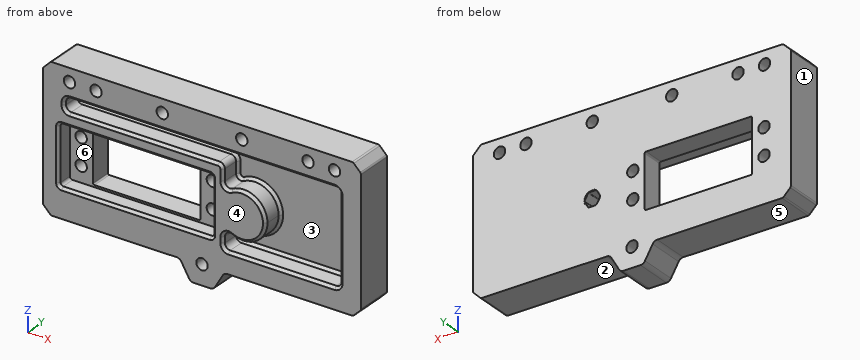
```python
from build123d import *

# Parameters (mm, degrees)
SKETCH_1_W          = 120
SKETCH_1_H          = 44
SKETCH_1_R          = 2.15
EXTRUDE_1_DEPTH     = 8
SKETCH_2_R          = 3
CUT_EXTRUDE_1_DEPTH = 0.1
MOVE_FACE_1_BY      = 10
EXTRUDE_START       = 6
SKETCH_3_W          = 120
SKETCH_3_H          = 54
SKETCH_3_W_2        = 58
SKETCH_3_H_2        = 22
EXTRUDE_2_DEPTH     = 6
SKETCH_4_R          = 2.15
CUT_EXTRUDE_2_DEPTH = 92.942930669
CUT_EXTRUDE_3_DEPTH = 8
FILLET_1_R          = 2
FILLET_2_R          = 2
FILLET_4_R          = 1
CHAMFER_1_SIZE      = 3
FILLET_5_R          = 1
SKETCH_6_R          = 2.15
EXTRUDE_3_DEPTH     = 14
SKETCH_6_3_R        = 2.15
CUT_EXTRUDE_6_DEPTH = 92.942930669
FILLET_6_R          = 2
CHAMFER_2_SIZE      = 1
SKETCH1_R           = 5.281314446
BOSS_EXTRUDE1_DEPTH = 4
SKETCH_7_R          = 2.15
CUT_EXTRUDE_7_DEPTH = 92.942930669


with BuildPart() as part:
    # 草图1 → 凸台-拉伸1 (new body)
    with BuildSketch(Plane(origin=(0, 0, 0), x_dir=(1, 0, 0), z_dir=(0, 1, 0))):
        with Locations((25.05, 0)):
            Rectangle(SKETCH_1_W, SKETCH_1_H)
        with Locations(Location((-24.75, 5, 0), (0, 0, 270))):
            Circle(SKETCH_1_R, mode=Mode.SUBTRACT)
        with Locations(Location((-24.75, -5, 0), (0, 0, 270))):
            Circle(SKETCH_1_R, mode=Mode.SUBTRACT)
        with Locations(Location((24.75, -5, 0), (0, 0, 270))):
            Circle(SKETCH_1_R, mode=Mode.SUBTRACT)
        with Locations(Location((24.75, 5, 0), (0, 0, 270))):
            Circle(SKETCH_1_R, mode=Mode.SUBTRACT)
        with BuildLine():
            Line((19.75, -10.25), (-19.75, -10.25))
            ThreePointArc((-19.75, -10.25), (-20.103553391, -10.103553391), (-20.25, -9.75))
            Line((-20.25, -9.75), (-20.25, 9.75))
            ThreePointArc((-20.25, 9.75), (-20.103553391, 10.103553391), (-19.75, 10.25))
            Line((-19.75, 10.25), (19.75, 10.25))
            ThreePointArc((19.75, 10.25), (20.103553391, 10.103553391), (20.25, 9.75))
            Line((20.25, 9.75), (20.25, -9.75))
            ThreePointArc((20.25, -9.75), (20.103553391, -10.103553391), (19.75, -10.25))
        make_face(mode=Mode.SUBTRACT)
        with BuildLine():
            Line((42.994486373, 0.15), (41.652146997, 2.475))
            ThreePointArc((41.652146997, 2.475), (41.542339376, 2.584807621), (41.392339376, 2.625))
            Line((41.392339376, 2.625), (38.707660624, 2.625))
            ThreePointArc((38.707660624, 2.625), (38.557660624, 2.584807621), (38.447853003, 2.475))
            Line((38.447853003, 2.475), (37.105513627, 0.15))
            ThreePointArc((37.105513627, 0.15), (37.065321248, 0), (37.105513627, -0.15))
            Line((37.105513627, -0.15), (38.447853003, -2.475))
            ThreePointArc((38.447853003, -2.475), (38.557660624, -2.584807621), (38.707660624, -2.625))
            Line((38.707660624, -2.625), (41.392339376, -2.625))
            ThreePointArc((41.392339376, -2.625), (41.542339376, -2.584807621), (41.652146997, -2.475))
            Line((41.652146997, -2.475), (42.994486373, -0.15))
            ThreePointArc((42.994486373, -0.15), (43.034678752, 0), (42.994486373, 0.15))
        make_face(mode=Mode.SUBTRACT)
    extrude(amount=EXTRUDE_1_DEPTH)

    # 草图2 → 切除-拉伸1 (cut)
    with BuildSketch(Plane(origin=(0, 8, 0), x_dir=(1, 0, 0), z_dir=(0, 1, 0))):
        with Locations(Location((40.05, 0, 0), (0, 0, 270))):
            Circle(SKETCH_2_R)
    extrude(amount=-CUT_EXTRUDE_1_DEPTH, mode=Mode.SUBTRACT)

    # Move Face 1: a face moved outward by 10.0
    extrude(part.faces().sort_by_distance((25.05, 4, 22))[0], amount=MOVE_FACE_1_BY, dir=(0, 0, 1))

    # 草图3 → 凸台-拉伸2 (add)
    with BuildSketch(Plane.XZ.offset(EXTRUDE_START)):
        with Locations((25.05, 5)):
            Rectangle(SKETCH_3_W, SKETCH_3_H)
        Rectangle(SKETCH_3_W_2, SKETCH_3_H_2, mode=Mode.SUBTRACT)
        with BuildLine():
            Line((41.652146997, 2.475), (42.994486373, 0.15))
            ThreePointArc((42.994486373, 0.15), (43.034678752, 0), (42.994486373, -0.15))
            Line((42.994486373, -0.15), (41.652146997, -2.475))
            ThreePointArc((41.652146997, -2.475), (41.542339376, -2.584807621), (41.392339376, -2.625))
            Line((41.392339376, -2.625), (38.707660624, -2.625))
            ThreePointArc((38.707660624, -2.625), (38.557660624, -2.584807621), (38.447853003, -2.475))
            Line((38.447853003, -2.475), (37.105513627, -0.15))
            ThreePointArc((37.105513627, -0.15), (37.065321248, 0), (37.105513627, 0.15))
            Line((37.105513627, 0.15), (38.447853003, 2.475))
            ThreePointArc((38.447853003, 2.475), (38.557660624, 2.584807621), (38.707660624, 2.625))
            Line((38.707660624, 2.625), (41.392339376, 2.625))
            ThreePointArc((41.392339376, 2.625), (41.542339376, 2.584807621), (41.652146997, 2.475))
        make_face(mode=Mode.SUBTRACT)
    extrude(amount=-EXTRUDE_2_DEPTH)

    # 草图4 → 切除-拉伸2 (cut, through all)
    with BuildSketch(Plane.XZ.offset(6)):
        with Locations(Location((-24.95, 27, 0), (0, 0, 270))):
            Circle(SKETCH_4_R)
        with Locations(Location((-14.95, 27, 0), (0, 0, 270))):
            Circle(SKETCH_4_R)
        with Locations(Location((65.05, 27, 0), (0, 0, 90))):
            Circle(SKETCH_4_R)
        with Locations(Location((75.05, 27, 0), (0, 0, 90))):
            Circle(SKETCH_4_R)
    extrude(amount=-CUT_EXTRUDE_2_DEPTH, mode=Mode.SUBTRACT)

    # 草图5 → 切除-拉伸3 (cut)
    with BuildSketch(Plane.XZ.offset(6)):
        with BuildLine():
            Line((59.05, 21), (-8.95, 21))
            Line((-8.95, 21), (-26.95, 21))
            Line((-26.95, 21), (-26.95, 16))
            Line((-26.95, 16), (33, 16))
            Line((33, 16), (33, 5.59441686))
            ThreePointArc((33, 5.59441686), (43.012262649, 8.498529285), (49.05, 0))
            ThreePointArc((49.05, 0), (43.012262649, -8.498529285), (33, -5.59441686))
            Line((33, -5.59441686), (33, -14))
            Line((33, -14), (77.05, -14))
            Line((77.05, -14), (77.05, 21))
            Line((77.05, 21), (59.05, 21))
        make_face()
    extrude(amount=-CUT_EXTRUDE_3_DEPTH, mode=Mode.SUBTRACT)

    # 圆角1
    fillet_1_edges = [part.edges().sort_by_distance(p)[0] for p in [
        (33, -2, 5.59441686),
        (33, -2, 16),
        (-26.95, -2, 16),
        (-26.95, -2, 21),
        (77.05, -2, 21),
        (77.05, -2, -14),
        (33, -2, -14),
    ]]
    fillet(fillet_1_edges, radius=FILLET_1_R)

    # 圆角2
    fillet_2_edges = [part.edges().sort_by_distance(p)[0] for p in [
        (33, -2, -5.59441686),
    ]]
    fillet(fillet_2_edges, radius=FILLET_2_R)

    # 圆角4
    fillet_4_edges = [part.edges().sort_by_distance(p)[0] for p in [
        (-29, -3, -11),
        (29, -3, -11),
        (29, -3, 11),
        (-29, -3, 11),
    ]]
    fillet(fillet_4_edges, radius=FILLET_4_R)

    # 倒角1
    chamfer_1_edges = [part.edges().sort_by_distance(p)[0] for p in [
        (-34.95, 1, -22),
        (85.05, 1, -22),
        (85.05, 1, 32),
        (-34.95, 1, 32),
    ]]
    chamfer(chamfer_1_edges, length=CHAMFER_1_SIZE)

    # 圆角5
    fillet_5_edges = [part.edges().sort_by_distance(p)[0] for p in [
        (85.05, 1, -19),
        (85.05, 1, 29),
        (-31.95, 1, 32),
        (82.05, 1, 32),
        (-31.95, 1, -22),
        (82.05, 1, -22),
        (-34.95, 1, -19),
        (-34.95, 1, 29),
    ]]
    fillet(fillet_5_edges, radius=FILLET_5_R)

    # 草图6 → 凸台-拉伸3 (add)
    with BuildSketch(Plane.XZ.offset(6)):
        Polygon((33.710254038, -21.5), (29.380127019, -14), (20.719872981, -14), (16.389745962, -21.5), (20.719872981, -29), (29.380127019, -29), align=None)
        with Locations((25.05, -21.5)):
            Circle(SKETCH_6_R, mode=Mode.SUBTRACT)
    extrude(amount=-EXTRUDE_3_DEPTH)

    # 草图6<3> → 切除-拉伸6 (cut, through all)
    with BuildSketch(Plane.XZ.offset(6)):
        with Locations(Location((25.05, -21.5, 0), (0, 0, 270))):
            Circle(SKETCH_6_3_R)
    extrude(amount=-CUT_EXTRUDE_6_DEPTH, mode=Mode.SUBTRACT)

    # 圆角6
    fillet_6_edges = [part.edges().sort_by_distance(p)[0] for p in [
        (16.678421097, 1, -22),
        (33.421578903, 1, -22),
        (20.719872981, 1, -29),
        (29.380127019, 1, -29),
    ]]
    fillet(fillet_6_edges, radius=FILLET_6_R)

    # 倒角2
    chamfer_2_edges = [part.edges().sort_by_distance(p)[0] for p in [
        (33, -6, 11.886141115),
        (33, 2, 11.886141115),
        (33, 2, -10.886141115),
        (55.025, 2, -14),
        (77.05, 2, 3.5),
        (25.05, 2, 21),
        (-26.95, 2, 18.5),
        (3.025, 2, 16),
        (33.585786438, 2, -13.414213562),
        (-26.364213562, 2, 20.414213562),
        (76.464213562, 2, -13.414213562),
        (76.464213562, 2, 20.414213562),
        (-26.364213562, 2, 16.585786438),
        (33.95989511, 2, 8.06401357),
        (3.025, -6, 16),
        (-26.95, -6, 18.5),
        (25.05, -6, 21),
        (77.05, -6, 3.5),
        (55.025, -6, -14),
        (33, -6, -10.886141115),
        (32.414213562, -6, 15.414213562),
        (33.95989511, -6, 8.06401357),
        (-26.364213562, -6, 16.585786438),
        (76.464213562, -6, 20.414213562),
        (76.464213562, -6, -13.414213562),
        (-26.364213562, -6, 20.414213562),
        (33.585786438, -6, -13.414213562),
        (32.414213562, 2, 15.414213562),
        (49.05, 2, 0),
        (49.05, -6, 0),
        (33.95989511, 2, -8.06401357),
        (33.95989511, -6, -8.06401357),
        (0, -6, -11),
        (29, -6, 0),
        (0, -6, 11),
        (-29, -6, 0),
        (28.707106781, -6, -10.707106781),
        (28.707106781, -6, 10.707106781),
        (-28.707106781, -6, -10.707106781),
        (-28.707106781, -6, 10.707106781),
    ]]
    chamfer(chamfer_2_edges, length=CHAMFER_2_SIZE)

    # Sketch1 → Boss-Extrude1 (add)
    with BuildSketch(Plane.XZ.offset(6)):
        with Locations((40.074190607, 0)):
            Circle(SKETCH1_R)
    extrude(amount=-BOSS_EXTRUDE1_DEPTH)

    # 草图7 → 切除-拉伸7 (cut, through all)
    with BuildSketch(Plane.XZ.offset(6)):
        with Locations(Location((10.05, 27, 0), (0, 0, 270))):
            Circle(SKETCH_7_R)
        with Locations(Location((40.05, 27, 0), (0, 0, 90))):
            Circle(SKETCH_7_R)
    extrude(amount=-CUT_EXTRUDE_7_DEPTH, mode=Mode.SUBTRACT)


solid = part.part
```
The listing builds one solid part. Answer for the finished solid, in the listing's coordinates (mm). Face numbers are marked on the shaded views. A direction names the side the tool comes from. Coordinates: 2 decimals unless noted, no trailing zeros. Loops run counter-clockwise (first coordinate to the right, second up) from the corner with the lowest first, then second, coordinate; pieces in that order, holes last. Notation, with made-up numbers: M 48.25,26.5 L 53.25,26.5 A17 ccw 53.25,40.5 Z; hole C 69,80 d3. An arc over 180 degrees is marked long. Answer as a JSON object with one key per item and string values. Group by question number.
Item 1: Which of the six approach directions +Z, -Z, +X, -X, +Y, -Y give full straight-line access (tool end or side, diameter ignored) to the marked faces 1, 2 and 3?
Item 2: Each of these flat-tipped pins is pushed along its axis until it touches: P1, Ø4, axis at x = 51, y = 2, coming from the -Z side; P2, Ø5.5, axis at x = 40.05, z = 27, coming from the +Y side; P3, Ø3, axis at x = 40, z = 0, coming from the +Y side; P4, Ø5, axis at x = -24.75, z = -5, coming from the -Y side. Where does it stop, or does it pass through?
Item 3: Section C-C (x = -8) is taken. Write down the section's boundary in (y, z), and give its area (3 significant figures).
Item 4: Consider L1, parallel to X at y = 5, z = -5; L2, parallel to Z at x = 75.05, y = -1; L3, parallel to X at y = -1, z = -9.5. Determine where each line is inside the solid, lowest interval first.
Item 5: Section D-D (z = 5) is taken. Give the number of separate pieces and of enclosed holes in the cut face, and give its area (3 significant figures).
Item 6: Section B-B (z = 27) is taken. Write down the section's boundary in (x, y), and give its area (3 significant figures).
Item 7: Determine the mould class of the marked faces 4, 5 and 6 for opening direction Z: +Z half, -Z half, draft (parallel to the pull), parting line (faces both ways), or undercut.
Solved:
{
 "1": {"face 1": "+Z, -Z, -X, +Y, -Y", "face 2": "-Z, +X, +Y, -Y", "face 3": "-Y"},
 "2": {"P1": "stops at z = -22", "P2": "stops at y = 8", "P3": "stops at y = -2", "P4": "stops at y = 0"},
 "3": {"outline": "M -6,-22 L 8,-22 L 8,-10.25 L 0,-10.25 L 0,-11 L -5,-11 L -6,-12 Z; M -6,12 L -5,11 L 0,11 L 0,10.25 L 8,10.25 L 8,32 L -6,32 L -6,22 L -5,21 L 1,21 L 2,20 L 2,17 L 1,16 L -5,16 L -6,15 Z", "area": "419 mm2"},
 "4": {"L1": "x = -34.95 to -26.9, -22.6 to -20.25, 20.25 to 22.6, 26.9 to 85.05", "L2": "z = -22 to -14, 21 to 24.85, 29.15 to 32", "L3": "x = -34.95 to -29, 29 to 33.02, 77.05 to 85.05"},
 "5": {"separate pieces": "4", "enclosed holes": "0", "area": "702 mm2"},
 "6": {"outline": "M -34.95,-6 L -27.1,-6 L -27.1,8 L -34.95,8 Z; M -22.8,-6 L -17.1,-6 L -17.1,8 L -22.8,8 Z; M -12.8,-6 L 7.9,-6 L 7.9,8 L -12.8,8 Z; M 12.2,-6 L 37.9,-6 L 37.9,8 L 12.2,8 Z; M 42.2,-6 L 62.9,-6 L 62.9,8 L 42.2,8 Z; M 67.2,-6 L 72.9,-6 L 72.9,8 L 67.2,8 Z; M 77.2,-6 L 85.05,-6 L 85.05,8 L 77.2,8 Z", "area": "1,320 mm2"},
 "7": {"face 4": "draft", "face 5": "-Z half", "face 6": "undercut"}
}
